Source: CAD feature listing. Evaluate the final solid. Frame: model axes, mm. Face numbers are marked on the shaded views. A direction names the side the tool comes from. Round coordinates to 2 decimals unless told otherwise and drop trailing zeros. Order: outer loops, then holes, each group sorted by start corner. A loop starts at its lowest first (then second) coordinate and runs counter-clockwise, first axis right, second up. Notation, with made-up numbers: (18, 78) -> (35, 78) arc R13 ccw to (35, 95) -> close; hole circle Ø4 at (10.5, -6). An arc over 180 degrees is marked (long way). Answer as CSV lines item,"result".
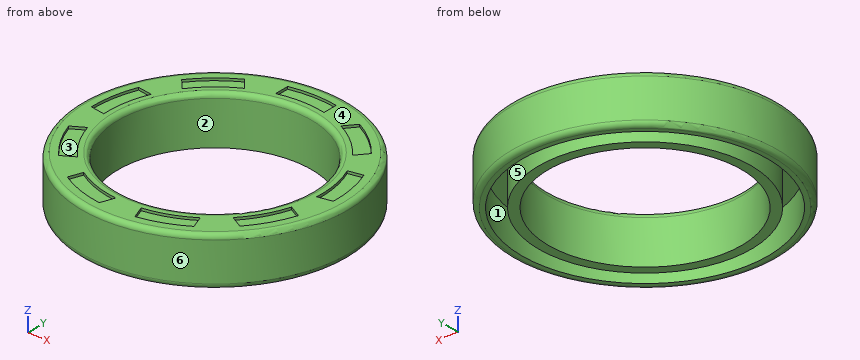
from build123d import *

# Parameters (mm, degrees)
SKETCH_1_R          = 27.5
EXTRUDE_1_DEPTH     = 10
SKETCH_2_R          = 20
CUT_EXTRUDE_1_DEPTH = 20
SKETCH_3_R          = 25.5
SKETCH_3_R_2        = 22
CUT_EXTRUDE_2_DEPTH = 7
FILLET_1_R          = 1
CUT_EXTRUDE_START   = -0.5
CUT_EXTRUDE_3_DEPTH = 0.5
FILLET_2_R          = 1


with BuildPart() as part:
    # 草图1 → 拉伸1 (new body)
    with BuildSketch(Plane.XY):
        Circle(SKETCH_1_R)
    extrude(amount=EXTRUDE_1_DEPTH)

    # 草图2 → 切除-拉伸1 (cut)
    with BuildSketch(Plane.XY.offset(10)):
        Circle(SKETCH_2_R)
    extrude(amount=-CUT_EXTRUDE_1_DEPTH, mode=Mode.SUBTRACT)

    # 草图3 → 切除-拉伸2 (cut)
    with BuildSketch(Plane(origin=(0, 0, 0), x_dir=(-1, 0, 0), z_dir=(0, 0, -1))):
        Circle(SKETCH_3_R)
        Circle(SKETCH_3_R_2, mode=Mode.SUBTRACT)
    extrude(amount=-CUT_EXTRUDE_2_DEPTH, mode=Mode.SUBTRACT)

    # 圆角1
    fillet_1_edges = [part.edges().sort_by_distance(p)[0] for p in [
        (-27.5, 0, 0),
        (-27.5, 0, 10),
    ]]
    fillet(fillet_1_edges, radius=FILLET_1_R)

    # 草图4 → 切除-拉伸3 (cut)
    with BuildSketch(Plane.XY.offset(10).offset(CUT_EXTRUDE_START)):
        with BuildLine():
            Line((17.601487344, 13.198016642), (19.575238783, 15.550242011))
            ThreePointArc((19.575238783, 15.550242011), (16.069690242, 19.151111078), (11.914794352, 21.978118108))
            Line((11.914794352, 21.978118108), (9.941042912, 19.625892739))
            ThreePointArc((9.941042912, 19.625892739), (14.141327413, 16.852977749), (17.601487344, 13.198016642))
        make_face()
        with BuildLine():
            Line((5, 21.424285286), (5, 24.494897428))
            ThreePointArc((5, 24.494897428), (0, 25), (-5, 24.494897428))
            Line((-5, 24.494897428), (-5, 21.424285286))
            ThreePointArc((-5, 21.424285286), (0, 22), (5, 21.424285286))
        make_face()
        with BuildLine():
            Line((21.96704314, -1.203750667), (24.991005785, -0.670544465))
            ThreePointArc((24.991005785, -0.670544465), (24.620193825, 4.341204442), (23.254524008, 9.177533066))
            Line((23.254524008, 9.177533066), (20.230561364, 8.644326863))
            ThreePointArc((20.230561364, 8.644326863), (21.665770566, 3.820259909), (21.96704314, -1.203750667))
        make_face()
        with BuildLine():
            Line((16.053975315, -15.042269662), (18.713203436, -16.577575733))
            ThreePointArc((18.713203436, -16.577575733), (21.650635095, -12.5), (23.713203436, -7.917321695))
            Line((23.713203436, -7.917321695), (21.053975315, -6.382015624))
            ThreePointArc((21.053975315, -6.382015624), (19.052558883, -11), (16.053975315, -15.042269662))
        make_face()
        with BuildLine():
            Line((2.62907402, -21.842343505), (3.679285225, -24.727775076))
            ThreePointArc((3.679285225, -24.727775076), (8.550503583, -23.49231552), (13.076211433, -21.307573643))
            Line((13.076211433, -21.307573643), (12.026000228, -18.422142072))
            ThreePointArc((12.026000228, -18.422142072), (7.524443153, -20.673237657), (2.62907402, -21.842343505))
        make_face()
        with BuildLine():
            Line((-12.026000228, -18.422142072), (-13.076211433, -21.307573643))
            ThreePointArc((-13.076211433, -21.307573643), (-8.550503583, -23.49231552), (-3.679285225, -24.727775076))
            Line((-3.679285225, -24.727775076), (-2.62907402, -21.842343505))
            ThreePointArc((-2.62907402, -21.842343505), (-7.524443153, -20.673237657), (-12.026000228, -18.422142072))
        make_face()
        with BuildLine():
            Line((-21.053975315, -6.382015624), (-23.713203436, -7.917321695))
            ThreePointArc((-23.713203436, -7.917321695), (-21.650635095, -12.5), (-18.713203436, -16.577575733))
            Line((-18.713203436, -16.577575733), (-16.053975315, -15.042269662))
            ThreePointArc((-16.053975315, -15.042269662), (-19.052558883, -11), (-21.053975315, -6.382015624))
        make_face()
        with BuildLine():
            Line((-20.230561364, 8.644326863), (-23.254524008, 9.177533066))
            ThreePointArc((-23.254524008, 9.177533066), (-24.620193825, 4.341204442), (-24.991005785, -0.670544465))
            Line((-24.991005785, -0.670544465), (-21.96704314, -1.203750667))
            ThreePointArc((-21.96704314, -1.203750667), (-21.665770566, 3.820259909), (-20.230561364, 8.644326863))
        make_face()
        with BuildLine():
            Line((-9.941042912, 19.625892739), (-11.914794352, 21.978118108))
            ThreePointArc((-11.914794352, 21.978118108), (-16.069690242, 19.151111078), (-19.575238783, 15.550242011))
            Line((-19.575238783, 15.550242011), (-17.601487344, 13.198016642))
            ThreePointArc((-17.601487344, 13.198016642), (-14.141327413, 16.852977749), (-9.941042912, 19.625892739))
        make_face()
    extrude(amount=CUT_EXTRUDE_3_DEPTH, mode=Mode.SUBTRACT)

    # 圆角2
    fillet_2_edges = [part.edges().sort_by_distance(p)[0] for p in [
        (-20, 0, 10),
    ]]
    fillet(fillet_2_edges, radius=FILLET_2_R)


solid = part.part
1. Pin query (flat end, axial travel): pin 1 (1.4 mm diameter, centred on x = -23.5, y = 5, fed in from +Z); pin 2 (1.8 mm diameter, centred on x = -1.5, y = 22.5, fed in from +Z); pin 3 (1 mm diameter, centred on x = 16.5, z = 2.5, fed in from +Y); pin 4 (5 mm diameter, centred on x = 15.5, z = 6, fed in from -Y). Return the tip coordinate at first contact, or that it passes through.
Results below:
pin 1,"z = 9.5"
pin 2,"z = 10"
pin 3,"y = 22.37"
pin 4,"y = -24.23"
2. Line query: L1, parallel to Y at x = 0, z = 2; L2, parallel to Y at x = -15, z = 3; L3, parallel to X at y = -11, z = 0.5. Output: solid intervals per line, ascending. Write a range as [from, to].
Results below:
L1,"[-27.5, -25.5], [-22, -20], [20, 22], [25.5, 27.5]"
L2,"[-23.05, -20.62], [-16.09, -13.23], [13.23, 16.09], [20.62, 23.05]"
L3,"[-25.06, -23.01], [-19.05, -16.7], [16.7, 19.05], [23.01, 25.06]"
3. Mould query, pull axis X, two halves, no side actions, for the marked faces 4, 5 and 6. Classes: released by +X, released by -X, zero draft, split by the parting line, or undercut.
Results below:
face 4,"zero draft"
face 5,"undercut"
face 6,"split by the parting line"
4. Section query B-B on x = 0. Return loops of the section in (y, z), and give its area (3 significant figures).
Results below:
outline,"(-27.5, 1) arc R1 ccw to (-26.5, 0) -> (-25.5, 0) -> (-25.5, 7) -> (-22, 7) -> (-22, 0) -> (-20, 0) -> (-20, 9) arc R1 ccw to (-21, 10) -> (-26.5, 10) arc R1 ccw to (-27.5, 9) -> close; (20, 0) -> (22, 0) -> (22, 7) -> (25.5, 7) -> (25.5, 0) -> (26.5, 0) arc R1 ccw to (27.5, 1) -> (27.5, 9) arc R1 ccw to (26.5, 10) -> (25, 10) -> (25, 9.5) -> (22, 9.5) -> (22, 10) -> (21, 10) arc R1 ccw to (20, 9) -> close"
area,"98.2 mm2"
5. Section query C-C on z = 1.75. Return loops of the section in (x, y).
Results below:
outline,"circle Ø55 at (0, 0); circle Ø44 at (0, 0); hole circle Ø51 at (0, 0); hole circle Ø40 at (0, 0)"
6. Reachability of the marked faces 1, 2 and 3 from +Z, -Z, +X, -X, +Y, -Y: full face, straight path, thin tool, end or side. Return the list, or none.
Results below:
face 1,"-Z"
face 2,"+Z, -Z"
face 3,"+Z"
